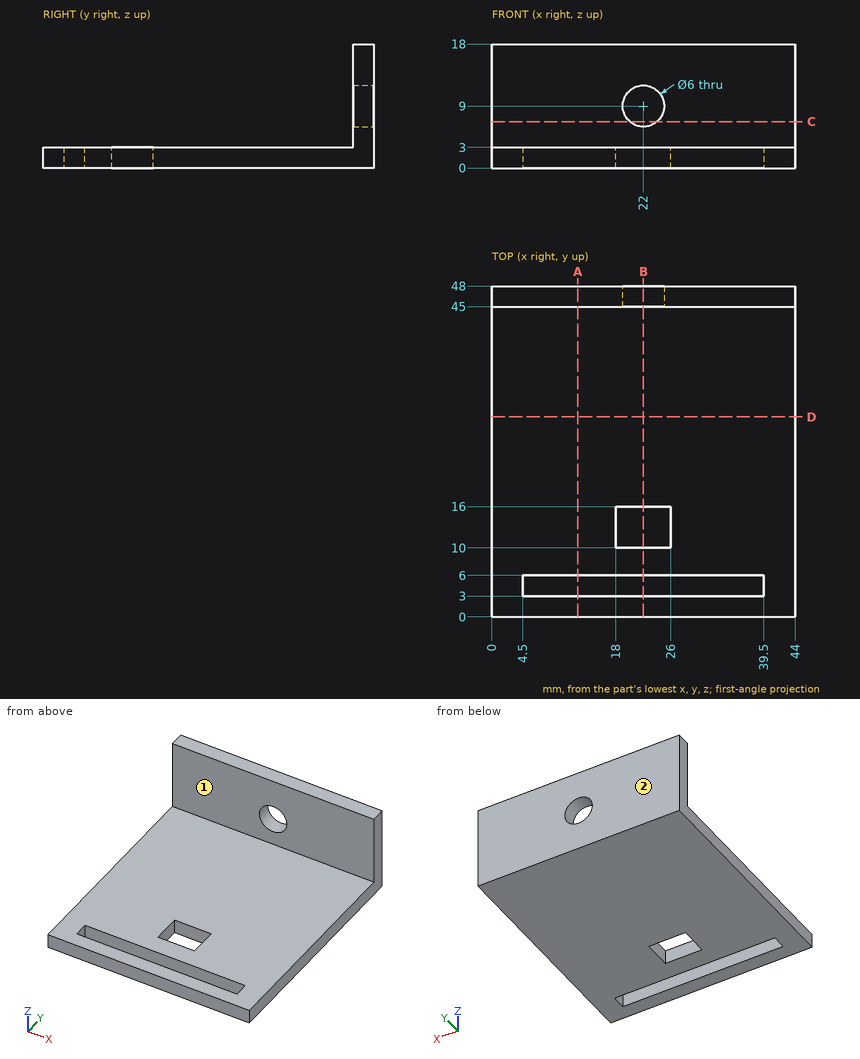
Print and shaded views of the part. All mm, measured from the part's lowest x, y and z. A direction names the side the tool comes from. Round coordinates to 2 decimals unless told otherwise and drop trailing zeros. Write each loop counter-clockwise with the first axis right and the second up, starting at its lowest first coordinate (ties: lowest second). Pieces come first, ordered by that corner, then holes. Notation, with made-up numbers: (80, 55) - (100, 55) arc R28 cw to (100, 77) - close; hole circle Ø6 at (-8, 6). An arc over 180 degrees is marked (long way). Use CSV: the item, a comma, the result in double quotes. Start each with the question number.
Item 1: Band-saw the part on C-C (z = 6.75). Write the cut outline in (x, y), and give its area (3 significant figures).
Item 2: Drill centre lines: L1, parallel to Z at x = 22, y = 46.85; L2, parallel to X at y = 46.55, z = 9; L3, parallel to X at y = 11, z = 2. Where is each one in solid material? Low to high. Write a range as [from, to].
Item 3: Tool access for the marked faces 1 and 2: list every direction of +Z, -Z, +X, -X, +Y, -Y with a clear straight run to the whole face (end or side of a thin tool).
Item 4: Pin check, flat tips, straight feed: P1, Ø1, axis at x = 8, y = 16.5, coming from the +Z side; P2, Ø8, axis at x = 39.5, z = 9.5, coming from the -Y side. Stop position of each tip, or through.
Item 5: Band-saw the part on B-B (x = 22). Write the cut outline in (y, z).
Item 6: Band-saw the part on D-D (y = 29). Write the cut outline in (x, z).
Item 7: Band-saw the part on A-A (x = 12.5). Write the cut outline in (y, z).
Checked values:
1,outline,"(0, 45) - (20.02, 45) - (20.02, 48) - (0, 48) - close; (23.98, 45) - (44, 45) - (44, 48) - (23.98, 48) - close"
1,area,"120 mm²"
2,L1,"z = [0, 6], [12, 18]"
2,L2,"x = [0, 19], [25, 44]"
2,L3,"x = [0, 18], [26, 44]"
3,face 1,"+Z, +X, -X, -Y"
3,face 2,"+Z, -Z, +X, -X, +Y"
4,P1,"stops at z = 3"
4,P2,"stops at y = 45"
5,outline,"(0, 0) - (3, 0) - (3, 3) - (0, 3) - close; (6, 0) - (10, 0) - (10, 3) - (6, 3) - close; (16, 0) - (48, 0) - (48, 6) - (45, 6) - (45, 3) - (16, 3) - close; (45, 12) - (48, 12) - (48, 18) - (45, 18) - close"
6,outline,"(0, 0) - (44, 0) - (44, 3) - (0, 3) - close"
7,outline,"(0, 0) - (3, 0) - (3, 3) - (0, 3) - close; (6, 0) - (48, 0) - (48, 18) - (45, 18) - (45, 3) - (6, 3) - close"
